Here's how the part is built. I have some questions about the finished solid (model axes, mm). A direction names the side the tool comes from. Coordinates: 2 decimals unless noted, no trailing zeros. Write each loop counter-clockwise with the first axis right and the second up, starting at its lowest first coordinate (ties: lowest second). Pieces come first, ordered by that corner, then holes.
from build123d import *

# Parameters (mm, degrees)
F2_R = 2.54


with BuildPart() as f1:
    # F0 (on Front) → F1 (revolve)
    with BuildSketch(Plane.XZ):
        with BuildLine():
            Line((0, 40.132), (0, 87.3506))
            ThreePointArc((0, 87.3506), (-4.7199768273, 88.1681648836), (-8.89, 90.5256))
            Line((-8.89, 90.5256), (-6.5449999258, 81.7739405792))
            add(Edge.make_bspline(
                [(-6.5449999258, 81.7739405792), (-10.5023747002, 71.8176961368), (-3.81, 66.0219296347)],
                knots=[1.0331645714, 1.0331645714, 1.0331645714, 2.617993878, 2.617993878, 2.617993878], degree=2, weights=[1, 0.7021280086, 1]))
            ThreePointArc((-3.81, 66.0219296347), (-11.1405483174, 60.0042932836), (-12.2581887711, 50.5862379799))
            ThreePointArc((-12.2581887711, 50.5862379799), (-10.7830325107, 26.1694758028), (-19.1262, 3.175))
            Line((-19.1262, 3.175), (-19.1262, 0))
            Line((-19.1262, 0), (-11.176, 0))
            Line((-11.176, 0), (-11.176, 8.509))
            Line((-11.176, 8.509), (-6.604, 13.081))
            Line((-6.604, 13.081), (-6.604, 33.528))
            Line((-6.604, 33.528), (0, 40.132))
        make_face()
    revolve(axis=Axis((0, 0, 63.7413), (0, 0, -1)))

    # F2
    f2_edges = [f1.edges().sort_by_distance(p)[0] for p in [
        (3.81, 0, 66.02193),
    ]]
    fillet(f2_edges, radius=F2_R)


solid = f1.part
1. Thinking about a two-plate mould opening in X: for faces 3 (the face through (-18.243, 5.745, 1.565)), 4 (the face through (8.87, -6.8, 4.31)), 5 (the face through (-6.1, -2.53, 23.45)), 6 (the face through (-8.2, -8.2, 0)), which applies, pulls with the +X half, pulls with the -X half, needs draft (parallel to the pull), parting line crosses it, or undercut?
2. If I drill on line 1 (X direction, y = 2.5, z = 20); line 2 (Z direction, x = 5, y = -2.5); line 3 (Y direction, x = 0, z = 5), over which ranges is the centre line in solid material (lowest first)?
3. I want a section at A-A (z = 24.5). List the corners of the cut face in (x, y) for me.
4. For pin 1 Ø8 at (x, y) = (12, -14.5) entering from -Z; pin 2 Ø15 at (x, y) = (0, 0) entering from +Z; pin 3 Ø10 at (y, z) = (-9.5, 37) entering from -X; pin 4 Ø12 at (x, z) = (-4.5, 64) entering from -Y, each with a flat end and sliding along its axis, tell me the tip position at first contact or that it passes through.
5. On a 3-axis mill with a long thin cutter (end or side, diameter ignored), from which of +Z, -Z, +X, -X, +Y, -Y can I reach the whole of each face in a straight line? I mean faces 1 (the face through (0.39, -1.75, 38.34)), 2 (the face through (5.698, -4.369, 84.144)). Say none if no direction works.
Response values:
1. face 3: parting line crosses it
1. face 4: undercut
1. face 5: undercut
1. face 6: needs draft
2. line 1: x = -11.75 to -6.11, 6.11 to 11.75
2. line 2: z = 34.54 to 65.8, 68.14 to 88.51
2. line 3: y = -18.05 to -11.18, 11.18 to 18.05
3. outline: circle Ø22.1 at (0, 0); hole circle Ø13.21 at (0, 0)
4. pin 1: stops at z = 0
4. pin 2: stops at z = 89.52
4. pin 3: stops at x = -9.16
4. pin 4: stops at y = -11.65
5. face 1: -Z
5. face 2: none
